Geometry check sheet. Reference: the model listing, model coordinates, mm. Face numbers are marked on the shaded views. Coordinates: 2 decimals unless noted, no trailing zeros. Write each loop counter-clockwise with the first axis right and the second up, starting at its lowest first coordinate (ties: lowest second). Pieces come first, ordered by that corner, then holes. Notation, with made-up numbers: (-30.5, -3.75) -> (-17.5, -3.75) arc R17 cw to (-17.5, 26.25) -> close; hole circle Ø6 at (-27.75, -2). An arc over 180 degrees is marked (long way). Use a Markdown table: item, result.
```python
from build123d import *

# Parameters (mm, degrees)
SKETCH1_R                = 60
BOSS_EXTRUDE1_DEPTH      = 140
SKETCH2_R                = 120
BOSS_EXTRUDE2_DEPTH      = 5
CHAMFER1_SIZE            = 2
SKETCH3_R                = 2.5
CUT_EXTRUDE1_DEPTH       = 332.700165812
CIRPATTERN1_COUNT        = 16
FILLET1_R                = 3
MIRROR1_COPY_1_SKETCH_R  = 2.5
MIRROR1_COPY_1_DEPTH     = 332.700165812
MIRROR1_COPY_2_SKETCH_R  = 2.5
MIRROR1_COPY_2_DEPTH     = 332.700165812
MIRROR1_COPY_3_SKETCH_R  = 2.5
MIRROR1_COPY_3_DEPTH     = 332.700165812
MIRROR1_COPY_4_SKETCH_R  = 2.5
MIRROR1_COPY_4_DEPTH     = 332.700165812
MIRROR1_COPY_5_SKETCH_R  = 2.5
MIRROR1_COPY_5_DEPTH     = 332.700165812
MIRROR1_COPY_6_SKETCH_R  = 2.5
MIRROR1_COPY_6_DEPTH     = 332.700165812
MIRROR1_COPY_7_SKETCH_R  = 2.5
MIRROR1_COPY_7_DEPTH     = 332.700165812
MIRROR1_COPY_8_SKETCH_R  = 2.5
MIRROR1_COPY_8_DEPTH     = 332.700165812
MIRROR1_COPY_9_SKETCH_R  = 2.5
MIRROR1_COPY_9_DEPTH     = 332.700165812
MIRROR1_COPY_10_SKETCH_R = 2.5
MIRROR1_COPY_10_DEPTH    = 332.700165812
MIRROR1_COPY_11_SKETCH_R = 2.5
MIRROR1_COPY_11_DEPTH    = 332.700165812
MIRROR1_COPY_12_SKETCH_R = 2.5
MIRROR1_COPY_12_DEPTH    = 332.700165812
MIRROR1_COPY_13_SKETCH_R = 2.5
MIRROR1_COPY_13_DEPTH    = 332.700165812
MIRROR1_COPY_14_SKETCH_R = 2.5
MIRROR1_COPY_14_DEPTH    = 332.700165812
MIRROR1_COPY_15_SKETCH_R = 2.5
MIRROR1_COPY_15_DEPTH    = 332.700165812
CHAMFER1_OF_MIRROR1_SIZE = 2
FILLET1_OF_MIRROR1_R     = 3


with BuildPart() as part:
    # Sketch1 → Boss-Extrude1 (new, symmetric)
    with BuildSketch(Plane.XY):
        Circle(SKETCH1_R)
    extrude(amount=BOSS_EXTRUDE1_DEPTH, both=True)

    # Sketch2 → Boss-Extrude2 (add)
    with BuildSketch(Plane.XY.offset(140)):
        Circle(SKETCH2_R)
    boss_extrude2 = extrude(amount=BOSS_EXTRUDE2_DEPTH)

    # Chamfer1
    chamfer1_edges = [part.edges().sort_by_distance(p)[0] for p in [
        (-120, 0, 140),
        (-120, 0, 145),
    ]]
    chamfer(chamfer1_edges, length=CHAMFER1_SIZE)

    # Sketch3 → Cut-Extrude1 (cut, through all)
    with BuildSketch(Plane.XY.offset(145)):
        with Locations((0, 90)):
            Circle(SKETCH3_R)
    cut_extrude1 = extrude(amount=-CUT_EXTRUDE1_DEPTH, mode=Mode.SUBTRACT)

    # CirPattern1: Cut-Extrude1 ×16 about axis
    cirpattern1_axis = Axis((0, 0, 140), (0, 0, 1))
    for i in range(1, CIRPATTERN1_COUNT):
        add(cut_extrude1.rotate(cirpattern1_axis, i * 360 / CIRPATTERN1_COUNT), mode=Mode.SUBTRACT)

    # Fillet1
    fillet1_edges = [part.edges().sort_by_distance(p)[0] for p in [
        (-60, 0, 140),
    ]]
    fillet(fillet1_edges, radius=FILLET1_R)

    # Sketch7 → CBORE for #12 Binding Head Machine Screw1 (revolve, cut)
    with BuildSketch(Plane(origin=(0, 0, 145), x_dir=(0, -1, 0), z_dir=(1, 0, 0))):
        Polygon((0, 0), (0, 290), (2.8956, 290), (2.8956, 3.5814), (5.95376, 3.5814), (5.95376, 0.532828266), (6.58876, 0), align=None)
    cbore_for_12_binding_head_machine_screw = revolve(axis=Axis((0, 0, 151.35), (0, 0, -1)), mode=Mode.SUBTRACT)

    # Mirror1: Boss-Extrude2, Cut-Extrude1, CBORE for #12 Binding Head Machine Screw1 across plane
    add(boss_extrude2.mirror(Plane.XY))
    add(cut_extrude1.mirror(Plane.XY), mode=Mode.SUBTRACT)
    add(cbore_for_12_binding_head_machine_screw.mirror(Plane.XY), mode=Mode.SUBTRACT)

    # Mirror1 copy 1 sketch → Mirror1 copy 1 (cut, through all)
    with BuildSketch(Plane(origin=(0, 0, -145), x_dir=(0.9238795325112867, 0.3826834323650898, 0), z_dir=(0, 0, -1))):
        with Locations((0, -90)):
            Circle(MIRROR1_COPY_1_SKETCH_R)
    extrude(amount=-MIRROR1_COPY_1_DEPTH, mode=Mode.SUBTRACT)

    # Mirror1 copy 2 sketch → Mirror1 copy 2 (cut, through all)
    with BuildSketch(Plane(origin=(0, 0, -145), x_dir=(0.7071067811865476, 0.7071067811865475, 0), z_dir=(0, 0, -1))):
        with Locations((0, -90)):
            Circle(MIRROR1_COPY_2_SKETCH_R)
    extrude(amount=-MIRROR1_COPY_2_DEPTH, mode=Mode.SUBTRACT)

    # Mirror1 copy 3 sketch → Mirror1 copy 3 (cut, through all)
    with BuildSketch(Plane(origin=(0, 0, -145), x_dir=(0.38268343236508984, 0.9238795325112867, 0), z_dir=(0, 0, -1))):
        with Locations((0, -90)):
            Circle(MIRROR1_COPY_3_SKETCH_R)
    extrude(amount=-MIRROR1_COPY_3_DEPTH, mode=Mode.SUBTRACT)

    # Mirror1 copy 4 sketch → Mirror1 copy 4 (cut, through all)
    with BuildSketch(Plane.YX.offset(145)):
        with Locations((0, -90)):
            Circle(MIRROR1_COPY_4_SKETCH_R)
    extrude(amount=-MIRROR1_COPY_4_DEPTH, mode=Mode.SUBTRACT)

    # Mirror1 copy 5 sketch → Mirror1 copy 5 (cut, through all)
    with BuildSketch(Plane(origin=(0, 0, -145), x_dir=(-0.3826834323650897, 0.9238795325112867, 0), z_dir=(0, 0, -1))):
        with Locations((0, -90)):
            Circle(MIRROR1_COPY_5_SKETCH_R)
    extrude(amount=-MIRROR1_COPY_5_DEPTH, mode=Mode.SUBTRACT)

    # Mirror1 copy 6 sketch → Mirror1 copy 6 (cut, through all)
    with BuildSketch(Plane(origin=(0, 0, -145), x_dir=(-0.7071067811865475, 0.7071067811865476, 0), z_dir=(0, 0, -1))):
        with Locations((0, -90)):
            Circle(MIRROR1_COPY_6_SKETCH_R)
    extrude(amount=-MIRROR1_COPY_6_DEPTH, mode=Mode.SUBTRACT)

    # Mirror1 copy 7 sketch → Mirror1 copy 7 (cut, through all)
    with BuildSketch(Plane(origin=(0, 0, -145), x_dir=(-0.9238795325112867, 0.3826834323650899, 0), z_dir=(0, 0, -1))):
        with Locations((0, -90)):
            Circle(MIRROR1_COPY_7_SKETCH_R)
    extrude(amount=-MIRROR1_COPY_7_DEPTH, mode=Mode.SUBTRACT)

    # Mirror1 copy 8 sketch → Mirror1 copy 8 (cut, through all)
    with BuildSketch(Plane(origin=(0, 0, -145), x_dir=(-1, 0, 0), z_dir=(0, 0, -1))):
        with Locations((0, -90)):
            Circle(MIRROR1_COPY_8_SKETCH_R)
    extrude(amount=-MIRROR1_COPY_8_DEPTH, mode=Mode.SUBTRACT)

    # Mirror1 copy 9 sketch → Mirror1 copy 9 (cut, through all)
    with BuildSketch(Plane(origin=(0, 0, -145), x_dir=(-0.9238795325112868, -0.38268343236508967, 0), z_dir=(0, 0, -1))):
        with Locations((0, -90)):
            Circle(MIRROR1_COPY_9_SKETCH_R)
    extrude(amount=-MIRROR1_COPY_9_DEPTH, mode=Mode.SUBTRACT)

    # Mirror1 copy 10 sketch → Mirror1 copy 10 (cut, through all)
    with BuildSketch(Plane(origin=(0, 0, -145), x_dir=(-0.7071067811865477, -0.7071067811865475, 0), z_dir=(0, 0, -1))):
        with Locations((0, -90)):
            Circle(MIRROR1_COPY_10_SKETCH_R)
    extrude(amount=-MIRROR1_COPY_10_DEPTH, mode=Mode.SUBTRACT)

    # Mirror1 copy 11 sketch → Mirror1 copy 11 (cut, through all)
    with BuildSketch(Plane(origin=(0, 0, -145), x_dir=(-0.3826834323650895, -0.9238795325112868, 0), z_dir=(0, 0, -1))):
        with Locations((0, -90)):
            Circle(MIRROR1_COPY_11_SKETCH_R)
    extrude(amount=-MIRROR1_COPY_11_DEPTH, mode=Mode.SUBTRACT)

    # Mirror1 copy 12 sketch → Mirror1 copy 12 (cut, through all)
    with BuildSketch(Plane(origin=(0, 0, -145), x_dir=(0, -1, 0), z_dir=(0, 0, -1))):
        with Locations((0, -90)):
            Circle(MIRROR1_COPY_12_SKETCH_R)
    extrude(amount=-MIRROR1_COPY_12_DEPTH, mode=Mode.SUBTRACT)

    # Mirror1 copy 13 sketch → Mirror1 copy 13 (cut, through all)
    with BuildSketch(Plane(origin=(0, 0, -145), x_dir=(0.38268343236509, -0.9238795325112866, 0), z_dir=(0, 0, -1))):
        with Locations((0, -90)):
            Circle(MIRROR1_COPY_13_SKETCH_R)
    extrude(amount=-MIRROR1_COPY_13_DEPTH, mode=Mode.SUBTRACT)

    # Mirror1 copy 14 sketch → Mirror1 copy 14 (cut, through all)
    with BuildSketch(Plane(origin=(0, 0, -145), x_dir=(0.7071067811865474, -0.7071067811865477, 0), z_dir=(0, 0, -1))):
        with Locations((0, -90)):
            Circle(MIRROR1_COPY_14_SKETCH_R)
    extrude(amount=-MIRROR1_COPY_14_DEPTH, mode=Mode.SUBTRACT)

    # Mirror1 copy 15 sketch → Mirror1 copy 15 (cut, through all)
    with BuildSketch(Plane(origin=(0, 0, -145), x_dir=(0.9238795325112868, -0.38268343236508956, 0), z_dir=(0, 0, -1))):
        with Locations((0, -90)):
            Circle(MIRROR1_COPY_15_SKETCH_R)
    extrude(amount=-MIRROR1_COPY_15_DEPTH, mode=Mode.SUBTRACT)

    # Chamfer1 of Mirror1
    chamfer1_of_mirror1_edges = [part.edges().sort_by_distance(p)[0] for p in [
        (-120, 0, -140),
        (-120, 0, -145),
    ]]
    chamfer(chamfer1_of_mirror1_edges, length=CHAMFER1_OF_MIRROR1_SIZE)

    # Fillet1 of Mirror1
    fillet1_of_mirror1_edges = [part.edges().sort_by_distance(p)[0] for p in [
        (-60, 0, -140),
    ]]
    fillet(fillet1_of_mirror1_edges, radius=FILLET1_OF_MIRROR1_R)


solid = part.part
```
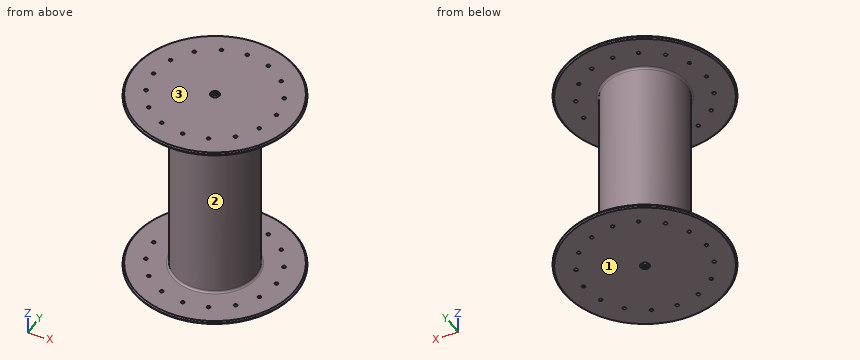
Item 1: Depth check by flat-ended pin: P1, Ø4, axis at x = 90, y = 0, coming from the +Z side; P2, Ø3, axis at y = -32, z = -91, coming from the -X side; P3, Ø3.5, axis at x = 2, y = -0.5, coming from the -Z side; P4, Ø12, axis at y = -21.5, z = -93.5, coming from the -X side. Enter the tip coordinate at first touch or a pass-through.
Answer block:
| item | result |
|---|---|
| P1 | passes through |
| P2 | stops at x = -51.67 |
| P3 | stops at z = -141.42 |
| P4 | stops at x = -57.96 |
Item 2: Thickness scan on L1, parallel to Z at x = 14, y = -91; L2, parallel to Y at x = 0, z = -38; L3, parallel to Z at x = -55.5, y = 28. Record the ranges inside material, lowest first. Write a range as [from, to].
Answer block:
| item | result |
|---|---|
| L1 | z = [-145, -140], [140, 145] |
| L2 | y = [-60, -2.9], [2.9, 60] |
| L3 | z = [-145, -139.88], [139.88, 145] |
Item 3: Mould release check, pull along Z, two halves, no side actions. Record for the marked faces 1, 2 and 3: +Z half, -Z half, draft (parallel to the pull), parting line (faces both ways), or undercut.
Answer block:
| item | result |
|---|---|
| face 1 | -Z half |
| face 2 | undercut |
| face 3 | +Z half |
Item 4: Section check A-A on z = -56. Record the boundary of the cut face in (x, y).
Answer block:
| item | result |
|---|---|
| outline | circle Ø120 at (0, 0); hole circle Ø5.79 at (0, 0) |
